Geometry check sheet. Reference: drawing and pictorial views, mm from the part's lowest x, y, z. A direction names the side the tool comes from. Coordinates: 2 decimals unless noted, no trailing zeros. Loops run counter-clockwise (first coordinate to the right, second up) from the corner with the lowest first, then second, coordinate; pieces in that order, holes last. Notation, with made-up numbers: (52.25, -15.75) -> (60.25, -15.75) arc R28 cw to (60.25, 8.25) -> close; hole circle Ø10 at (83, -4.5). An arc over 180 degrees is marked (long way). Answer as a JSON object with one key per item and string values.
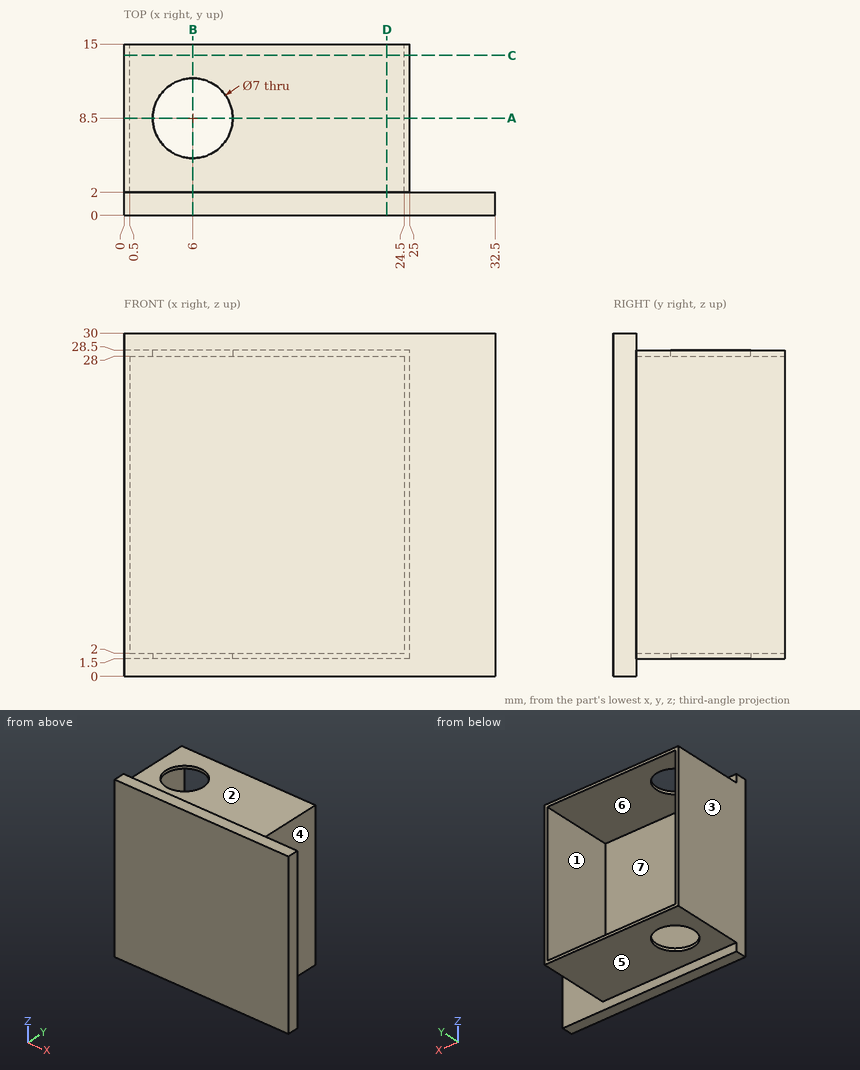
1. Thickness scan on probe 1 along X at (y, z) = (5.75, 10); probe 2 along Z at (x, y) = (22, 9.75); probe 3 along X at (y, z) = (8.5, 1.85). Record the ranges inside material, lowest first. Write a range as from..to.
Evaluation:
{"probe 1": "x = 0..0.5, 24.5..25", "probe 2": "z = 1.5..2, 28..28.5", "probe 3": "x = 0..2.5, 9.5..25"}
2. Section check D-D, the plane x = 23. Record the boundary of the cut face in (y, z), then the cut area to 3 significant figures.
Evaluation:
{"outline": "(0, 0) -> (2, 0) -> (2, 1.5) -> (15, 1.5) -> (15, 2) -> (2, 2) -> (2, 28) -> (15, 28) -> (15, 28.5) -> (2, 28.5) -> (2, 30) -> (0, 30) -> close", "area": "73.0 mm^2"}
3. Mould release check, pull along X, two halves, no side actions. Record for the marked faces 4, 5, 6 and 7: released by +X, released by -X, zero draft, split by the parting line, or undercut.
Evaluation:
{"face 4": "released by +X", "face 5": "zero draft", "face 6": "undercut", "face 7": "undercut"}
4. Section check C-C, the plane y = 14. Record the boundary of the cut face in (x, z).
Evaluation:
{"outline": "(0, 1.5) -> (25, 1.5) -> (25, 28.5) -> (0, 28.5) -> close; hole (0.5, 2) -> (24.5, 2) -> (24.5, 28) -> (0.5, 28) -> close"}
5. Section check B-B, the plane x = 6. Record the boundary of the cut face in (y, z).
Evaluation:
{"outline": "(0, 0) -> (2, 0) -> (2, 1.5) -> (5, 1.5) -> (5, 2) -> (2, 2) -> (2, 28) -> (5, 28) -> (5, 28.5) -> (2, 28.5) -> (2, 30) -> (0, 30) -> close; (12, 1.5) -> (15, 1.5) -> (15, 2) -> (12, 2) -> close; (12, 28) -> (15, 28) -> (15, 28.5) -> (12, 28.5) -> close"}
6. Section check A-A, the plane y = 8.5. Record the boundary of the cut face in (x, z).
Evaluation:
{"outline": "(0, 1.5) -> (2.5, 1.5) -> (2.5, 2) -> (0.5, 2) -> (0.5, 28) -> (2.5, 28) -> (2.5, 28.5) -> (0, 28.5) -> close; (9.5, 1.5) -> (25, 1.5) -> (25, 28.5) -> (9.5, 28.5) -> (9.5, 28) -> (24.5, 28) -> (24.5, 2) -> (9.5, 2) -> close"}
7. Depth check by flat-ended pin: P1, Ø4, axis at x = 7.5, y = 8, coming from the +Z side; P2, Ø12, axis at x = 9.5, z = 24.5, coming from the -Y side; P3, Ø4, axis at y = 9.5, z = 15, coming from the +X side; P4, Ø4, axis at x = 11.5, y = 6.5, coming from the -Z side. Enter the tip coordinate at first touch or a pass-through.
Evaluation:
{"P1": "stops at z = 28.5", "P2": "stops at y = 0", "P3": "stops at x = 25", "P4": "stops at z = 1.5"}
8. Tool access check on the marked faces 1, 2 and 3. Record the directions out of +Z, -Z, +X, -X, +Y, -Y that give a thin tool (end or side, any length) a straight path to the whole face; none if there is none.
Evaluation:
{"face 1": "+Y", "face 2": "+Z, +X, -X, +Y", "face 3": "+Z, -Z, -X, +Y, -Y"}
